Autodesk Inventor part; units mm, degrees
ref_plane "Work Plane1" through (0, 7, 5.75) normal (0, 0, 1) x (1, 0, 0)
ref_plane "YZ Plane" through (0, 0, 0) normal (1, 0, 0) x (0, 1, 0)
ref_plane "XZ Plane" through (0, 0, 0) normal (0, 1, 0) x (-1, 0, 0)
sketch "Sketch1" plane through (0, 0, 0) normal (0, 1, 0) x (-1, 0, 0)
  circle A0 centre (0, 0) radius 4
  dimension "d0" = 8
extrude "Extrusion1" add sketch "Sketch1" along normal blind 7
sketch "Sketch2" plane through (0, 7, 0) normal (0, 1, 0) x (1, 0, 0)
  circle A0 centre (0, 0) radius 5.75
  dimension "d3" = 11.5
extrude "Extrusion2" add sketch "Sketch2" along normal blind 3.2
sketch "Sketch4" plane through (0, 0, 0) normal (1, 0, 0) x (0, 1, 0)
  line L0 (20.4, 3.1121) -> (19.5121, 4)
  line L1 (19.5121, 4) -> (17.7879, 4)
  line L2 (16.9, 3.1121) -> (17.7879, 4)
  line L3 (13.4, 3.1121) -> (14.2879, 4)
  line L4 (14.2879, 4) -> (16.0121, 4)
  line L5 (16.9, 3.1121) -> (16.0121, 4)
  line L6 (13.4, 3.1121) -> (13.4, 6.6121)
  line L7 (13.4, 8.5445) -> (20.4, 8.5445)
  line L8 (20.4, 8.5445) -> (20.4, 3.1121)
  line L9 (0, 3.1121) -> (0.8879, 4)
  line L10 (0.8879, 4) -> (2.6121, 4)
  line L11 (3.5, 3.1121) -> (2.6121, 4)
  line L12 (3.5, 3.1121) -> (4.3879, 4)
  line L13 (6.1121, 4) -> (4.3879, 4)
  line L14 (7, 3.1121) -> (6.1121, 4)
  line L15 (7, 3.1121) -> (7, 6.6121)
  line L16 (7, 8.5445) -> (0, 8.5445)
  line L17 (0, 8.5445) -> (0, 3.1121)
  line L18 (13.4, 6.6121) -> (7, 6.6121)
  line L19 (13.4, 8.5445) -> (7, 8.5445)
  line L20 (-4.08, 0) -> (24.48, 0)
  point P0 (0, 0)
revolve "Revolution1" cut sketch "Sketch4" angle 360 about axis through (0, -10, 0) along (0, 1, 0)
hole "Hole2" at (0, 0, 0) direction (0, 1, 0) diameter 4.4 end through all
ref_plane "Work Plane1" through (0, 7, 5.75) normal (0, 0, 1) x (1, 0, 0)
sketch "Sketch5" plane through (0, 7, 5.75) normal (0, 0, 1) x (1, 0, 0)
  line L0 (5.75, 3.2) -> (-5.75, 3.2)
  line L1 (-5.75, 0) -> (5.75, 0)
  line L2 (-5.75, 0) -> (-5.75, 3.2)
  line L3 (5.75, 3.2) -> (5.75, 0)
  point P0 (0, -7)
extrude "Extrusion4" cut sketch "Sketch5" against normal through all
properties part number "M4-608 Straight Spacer"
CAD build for the part. Positions are in the model's coordinates, mm. Give positions to 0.01 mm unless a question says otherwise; leave off trailing zeros. Loops run counter-clockwise (first coordinate to the right, second up) from the corner with the lowest first, then second, coordinate; pieces in that order, holes last. Notation, with made-up numbers: (-15.75, -12.5) -> (-7.75, -12.5) arc R10 cw to (-7.75, -4.5) -> close; hole circle Ø1 at (-10.5, 57.5). An arc over 180 degrees is marked (long way). Use a Markdown table: item, result.
1. Slice it at C-C (y = 1). List the corners of the cut face in (x, z).
Check result:
| item | result |
|---|---|
| outline | circle Ø8 at (0, 0); hole circle Ø4.4 at (0, 0) |
2. Flat gauge pins, fed straight in: pin 1 (4 mm diameter, centred on y = 2.5, z = -1, fed in from +X); pin 2 (1 mm diameter, centred on x = 3, z = 3, fed in from -Y); pin 3 (1.5 mm diameter, centred on y = 1, z = 3, fed in from -X); pin 4 (4 mm diameter, centred on x = 3, y = 2.5, fed in from +Z). Where does each tip first touch, or does it go through?
Check result:
| item | result |
|---|---|
| pin 1 | stops at x = 4 |
| pin 2 | stops at y = 0.63 |
| pin 3 | stops at x = -3.31 |
| pin 4 | stops at z = 3.87 |
3. Slice it at D-D (y = 3.75). List the corners of the cut face in (x, z).
Check result:
| item | result |
|---|---|
| outline | circle Ø6.72 at (0, 0); hole circle Ø4.4 at (0, 0) |
4. Wall check: L1, parallel to X at y = 1.5, z = 0; L2, parallel to Y at x = 0, z = -3.5; L3, parallel to X at y = 4.25, z = 0. Give the ranges that are in metal, low to high. Write a range as [from, to].
Check result:
| item | result |
|---|---|
| L1 | x = [-4, -2.2], [2.2, 4] |
| L2 | y = [0.39, 3.11], [3.89, 6.61] |
| L3 | x = [-3.86, -2.2], [2.2, 3.86] |
5. Mould opens along X. For faces 1 (the cylindrical face through (0.867, 1.738, 3.905)), 2 (the flat face through (-2, 0, -1.3)), 3 (the cylindrical face through (-0.66, 3.55, -2.1)) say: pulls with the +X half, pulls with the -X half, needs draft (parallel to the pull), parting line crosses it, or undercut.
Check result:
| item | result |
|---|---|
| face 1 | parting line crosses it |
| face 2 | needs draft |
| face 3 | undercut |
6. Slice it at B-B (x = 0). List the corners of the cut face in (y, z), plus the area to 3 significant figures.
Check result:
| item | result |
|---|---|
| outline | (0, -3.11) -> (0.89, -4) -> (2.61, -4) -> (3.5, -3.11) -> (4.39, -4) -> (6.11, -4) -> (7, -3.11) -> (7, -2.2) -> (0, -2.2) -> close; (0, 2.2) -> (7, 2.2) -> (7, 3.11) -> (6.11, 4) -> (4.39, 4) -> (3.5, 3.11) -> (2.61, 4) -> (0.89, 4) -> (0, 3.11) -> close |
| area | 22.0 mm^2 |
7. Slice it at A-A (z = 0). List the corners of the cut face in (x, y), plus the area to 3 significant figures.
Check result:
| item | result |
|---|---|
| outline | (-4, 0.89) -> (-3.11, 0) -> (-2.2, 0) -> (-2.2, 7) -> (-3.11, 7) -> (-4, 6.11) -> (-4, 4.39) -> (-3.11, 3.5) -> (-4, 2.61) -> close; (2.2, 0) -> (3.11, 0) -> (4, 0.89) -> (4, 2.61) -> (3.11, 3.5) -> (4, 4.39) -> (4, 6.11) -> (3.11, 7) -> (2.2, 7) -> close |
| area | 22.0 mm^2 |
